Input: part model. Units: mm. Frame: model coordinates. Face numbers are marked on the shaded views. A direction names the side the tool comes from. Give positions to 0.01 mm unless a question says otherwise; leave off trailing zeros. Loops run counter-clockwise (first coordinate to the right, second up) from the corner with the lowest first, then second, coordinate; pieces in that order, holes last.
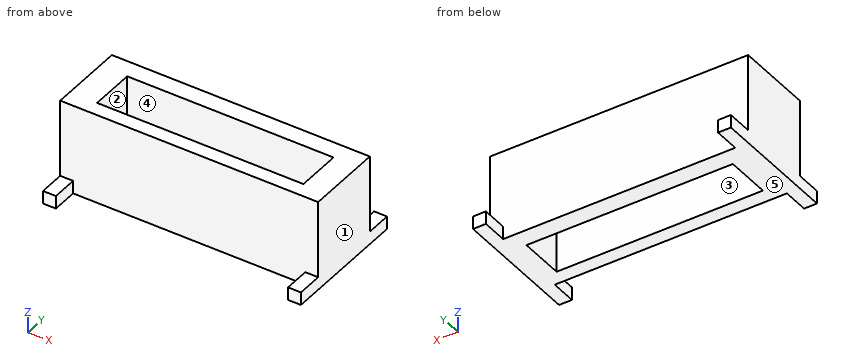
from build123d import *

# Parameters (mm, degrees)
BOX001_W     = 1
BOX001_H     = 10
BOX001_DEPTH = 1
BOX002_W     = 1
BOX002_H     = 10
BOX002_DEPTH = 1
BOX_W        = 20
BOX_H        = 6
BOX_DEPTH    = 7
SKETCH_W     = 16
SKETCH_H     = 3.5
POCKET_DEPTH = 9


with BuildPart() as cube001:
    # Box001 → Box001 (new body)
    with BuildSketch(Plane(origin=(0, -2, 0), x_dir=(1, 0, 0), z_dir=(0, 0, 1))):
        with Locations((0.5, 5)):
            Rectangle(BOX001_W, BOX001_H)
    extrude(amount=BOX001_DEPTH)


with BuildPart() as cube002:
    # Box002 → Box002 (new body)
    with BuildSketch(Plane(origin=(19, -2, 0), x_dir=(1, 0, 0), z_dir=(0, 0, 1))):
        with Locations((0.5, 5)):
            Rectangle(BOX002_W, BOX002_H)
    extrude(amount=BOX002_DEPTH)


with BuildPart() as fusion:
    # Box → Box (new body)
    with BuildSketch(Plane.XY):
        with Locations((10, 3)):
            Rectangle(BOX_W, BOX_H)
    extrude(amount=BOX_DEPTH)

    # Sketch (on Face6 of BaseFeature) → Pocket (cut)
    with BuildSketch(Plane.XY.offset(7)):
        with Locations((10.11532, 2.863184)):
            Rectangle(SKETCH_W, SKETCH_H)
    extrude(amount=-POCKET_DEPTH, mode=Mode.SUBTRACT)

    # Fusion: union Cube001, Cube002
    add(cube001.part)
    add(cube002.part)


solid = fusion.part
(1) Reachability of the marked faces 1 and 2 from +Z, -Z, +X, -X, +Y, -Y: full face, straight path, thin tool, end or side. Return the list, or none.
Values follow:
face 1: +Z, -Z, +X, +Y, -Y
face 2: +Z, -Z
(2) Ray query, probe 1 along Y at (x, z) = (17, 4.25); probe 2 along X at (y, z) = (3.75, 3.25); probe 3 along Y at (x, z) = (18.25, 2.75). Return the intervals inside material, ascending.
Values follow:
probe 1: y = 0 to 1.11, 4.61 to 6
probe 2: x = 0 to 2.12, 18.12 to 20
probe 3: y = 0 to 6
(3) Cut plane C-C (z = 4.75). Return the cut outline in (x, y).
Values follow:
outline: (0, 0) - (20, 0) - (20, 6) - (0, 6) - close; hole (2.12, 1.11) - (18.12, 1.11) - (18.12, 4.61) - (2.12, 4.61) - close
(4) Pin query (flat end, axial travel): pin 1 Ø1.1 at (x, y) = (19.5, -1) entering from +Z; pin 2 Ø3.5 at (x, z) = (8.5, 2) entering from -Y; pin 3 Ø3.5 at (x, z) = (9.5, 2) entering from +Y. Return the tip coordinate at first contact, or that it passes through.
Values follow:
pin 1: stops at z = 1
pin 2: stops at y = 0
pin 3: stops at y = 6
(5) Cut plane B-B (x = 14.25). Return the cut outline in (y, z).
Values follow:
outline: (0, 0) - (1.11, 0) - (1.11, 7) - (0, 7) - close; (4.61, 0) - (6, 0) - (6, 7) - (4.61, 7) - close
(6) Mould query, pull axis Y, two halves, no side actions, for the marked faces 3, 4 and 5. Classes: +Y half, -Y half, draft (parallel to the pull), parting line (faces both ways), or undercut.
Values follow:
face 3: undercut
face 4: undercut
face 5: draft
(7) Cut plane A-A (y = 2). Return the cut outline in (x, z).
Values follow:
outline: (0, 0) - (2.12, 0) - (2.12, 7) - (0, 7) - close; (18.12, 0) - (20, 0) - (20, 7) - (18.12, 7) - close
